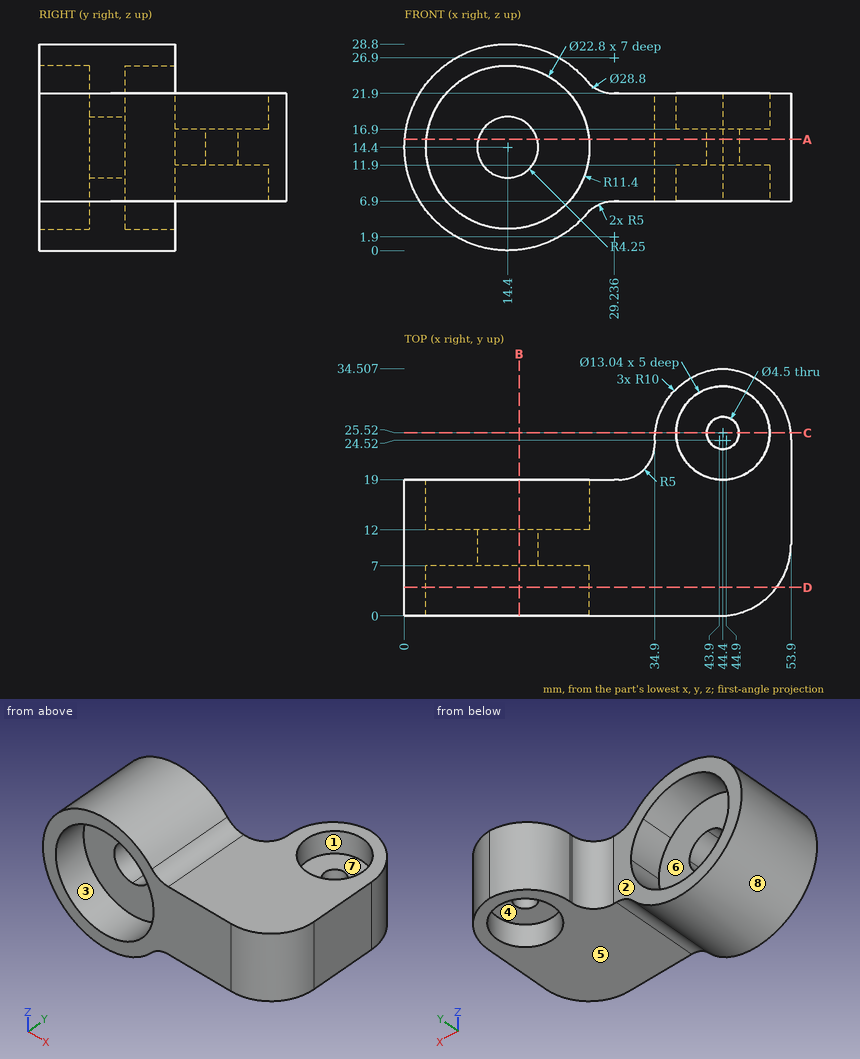
The drawing under review shows one solid part. Ordinate dimensions are in mm from its lowest x, y, z. A direction names the side the tool comes from. Give positions to 0.01 mm unless a question says otherwise; leave off trailing zeros. Write each loop counter-clockwise with the first axis right and the second up, starting at its lowest first coordinate (ties: lowest second). Pieces come first, ordered by that corner, then holes. Notation, with made-up numbers: (10.5, -37.75) - (58.5, -37.75) arc R10 ccw to (58.5, -30.75) - close; hole circle Ø1 at (71, 41). An arc over 180 degrees is marked (long way). Answer in a Markdown table with one row per item. Add a question column.
1. Tool access review of the marked faces 1, 2, 3, 4 and 5: name each direction out of +Z, -Z, +X, -X, +Y, -Y from which nothing blocks a thin tool from reaching the whole face with its end or side.
2. Draft analysis for pull direction Y (two halves, no side actions). For the marked faces 6, 7 and 8, state which applies: +Y half, -Y half, draft (parallel to the pull), parting line (faces both ways), or undercut.
3. We need section D-D on y = 4. Write out the cut boundary in (x, z).
4. We need section C-C on y = 25.52. Write out the cut boundary in (x, z).
5. Insertion check: P1, Ø15, axis at x = 44.4, y = 25.52, coming from the +Z side; P2, Ø1.5, axis at y = 5, z = 5, coming from the +X side (1 decimal); P3, Ø14.5, axis at x = 41.5, y = 24, coming from the -Z side; P4, Ø1, axis at x = 9.5, y = 21, coming from the -Z side. Each pin has a flat end and moves straight along its axis. Give the tip position at first contact, or say it passes through.
6. We need section B-B on x = 16. Write out the cut boundary in (y, z).
7. We need section A-A on z = 15.5. State how many separate pieces and enclosed holes the cut face has.
8. Wall thickness on line 1 along Y through (x, z) = (44.4, 10.35); line 2 along Y through (x, z) = (44.4, 15.4); line 3 along X through (y, z) = (16.25, 14.4): over which ranges is each line inside the solid? List them lowest first. Write a range as [from, to].
Ans:
| question | item | result |
|---|---|---|
| 1 | face 1 | +Z |
| 1 | face 2 | +Z, -Z, -X, +Y |
| 1 | face 3 | -Y |
| 1 | face 4 | -Z |
| 1 | face 5 | -Z, +X, +Y, -Y |
| 2 | face 6 | +Y half |
| 2 | face 7 | undercut |
| 2 | face 8 | draft |
| 3 | outline | (25.41, 5.12) arc R5 cw to (29.24, 6.9) - (51.9, 6.9) - (51.9, 21.9) - (29.24, 21.9) arc R5 cw to (25.41, 23.68) arc R14.4 ccw (long way) to start; hole circle Ø22.8 at (14.4, 14.4) |
| 4 | outline | (34.95, 6.9) - (37.88, 6.9) - (37.88, 11.9) - (42.15, 11.9) - (42.15, 16.9) - (37.88, 16.9) - (37.88, 21.9) - (34.95, 21.9) - close; (46.65, 11.9) - (50.92, 11.9) - (50.92, 6.9) - (53.85, 6.9) - (53.85, 21.9) - (50.92, 21.9) - (50.92, 16.9) - (46.65, 16.9) - close |
| 5 | P1 | stops at z = 21.9 |
| 5 | P2 | stops at x = 26 |
| 5 | P3 | stops at z = 6.9 |
| 5 | P4 | passes through |
| 6 | outline | (0, 0.09) - (19, 0.09) - (19, 3.11) - (12, 3.11) - (12, 10.46) - (7, 10.46) - (7, 3.11) - (0, 3.11) - close; (0, 25.69) - (7, 25.69) - (7, 18.34) - (12, 18.34) - (12, 25.69) - (19, 25.69) - (19, 28.71) - (0, 28.71) - close |
| 7 | separate pieces | 2 |
| 7 | enclosed holes | 1 |
| 8 | line 1 | y = [0.01, 19], [32.04, 34.51] |
| 8 | line 2 | y = [0.01, 23.27], [27.77, 34.51] |
| 8 | line 3 | x = [0, 3], [25.8, 53.9] |
